```python
from build123d import *

# Parameters (mm, degrees)
SKETCH1_R           = 2.54
BOSS_EXTRUDE1_DEPTH = 3.175
FILLET1_R           = 6.35
CUT_EXTRUDE1_DEPTH  = 342.972704503
FILLET2_R           = 3.175
SKETCH3_R           = 2.54
CUT_EXTRUDE2_DEPTH  = 342.972704503
FILLET3_R           = 1.5875


with BuildPart() as part:
    # Sketch1 → Boss-Extrude1 (new body)
    with BuildSketch(Plane.XY):
        Polygon((0, 25.4), (0, 0), (127, 0), (127, 25.4), (152.4, 88.9), (317.5, 88.9), (317.5, 127), (279.4, 127), (152.4, 127), (40.64, 127), align=None)
        with Locations((12.7, 12.7)):
            Circle(SKETCH1_R, mode=Mode.SUBTRACT)
        with Locations((63.5, 12.7)):
            Circle(SKETCH1_R, mode=Mode.SUBTRACT)
        with Locations((114.3, 12.7)):
            Circle(SKETCH1_R, mode=Mode.SUBTRACT)
        Polygon((302.262821178, 101.346), (306.075642355, 107.95), (302.262821178, 114.554), (294.637178822, 114.554), (290.824357645, 107.95), (294.637178822, 101.346), align=None, mode=Mode.SUBTRACT)
    extrude(amount=BOSS_EXTRUDE1_DEPTH)

    # Fillet1
    fillet1_edges = [part.edges().sort_by_distance(p)[0] for p in [
        (40.64, 127, 1.5875),
        (317.5, 127, 1.5875),
        (317.5, 88.9, 1.5875),
        (152.4, 88.9, 1.5875),
        (127, 25.4, 1.5875),
        (127, 0, 1.5875),
        (0, 0, 1.5875),
        (0, 25.4, 1.5875),
    ]]
    fillet(fillet1_edges, radius=FILLET1_R)

    # Sketch2 → Cut-Extrude1 (cut, through all)
    with BuildSketch(Plane.XY.offset(3.175)):
        Polygon((49.23831861, 114.3), (13.67831861, 25.4), (39.597669611, 25.4), (75.157669611, 114.3), align=None)
        Polygon((86.100324499, 114.3), (50.540324499, 25.4), (76.459675501, 25.4), (112.019675501, 114.3), align=None)
        Polygon((122.962330389, 114.3), (87.402330389, 25.4), (113.32168139, 25.4), (148.88168139, 114.3), align=None)
    extrude(amount=-CUT_EXTRUDE1_DEPTH, mode=Mode.SUBTRACT)

    # Fillet2
    fillet2_edges = [part.edges().sort_by_distance(p)[0] for p in [
        (76.459675501, 25.4, 1.5875),
        (50.540324499, 25.4, 1.5875),
        (86.100324499, 114.3, 1.5875),
        (112.019675501, 114.3, 1.5875),
        (148.88168139, 114.3, 1.5875),
        (113.32168139, 25.4, 1.5875),
        (87.402330389, 25.4, 1.5875),
        (122.962330389, 114.3, 1.5875),
        (39.597669611, 25.4, 1.5875),
        (13.67831861, 25.4, 1.5875),
        (49.23831861, 114.3, 1.5875),
        (75.157669611, 114.3, 1.5875),
    ]]
    fillet(fillet2_edges, radius=FILLET2_R)

    # Sketch3 → Cut-Extrude2 (cut, through all)
    with BuildSketch(Plane.XY.offset(3.175)):
        with Locations((45.72, 120.65)):
            Circle(SKETCH3_R)
        with Locations((119.38, 120.65)):
            Circle(SKETCH3_R)
        with Locations((193.04, 120.65)):
            Circle(SKETCH3_R)
        with Locations((266.7, 120.65)):
            Circle(SKETCH3_R)
    extrude(amount=-CUT_EXTRUDE2_DEPTH, mode=Mode.SUBTRACT)

    # Fillet3
    fillet3_edges = [part.edges().sort_by_distance(p)[0] for p in [
        (294.637178822, 101.346, 1.5875),
        (302.262821178, 101.346, 1.5875),
        (306.075642355, 107.95, 1.5875),
        (302.262821178, 114.554, 1.5875),
        (294.637178822, 114.554, 1.5875),
        (290.824357645, 107.95, 1.5875),
    ]]
    fillet(fillet3_edges, radius=FILLET3_R)


solid = part.part
```
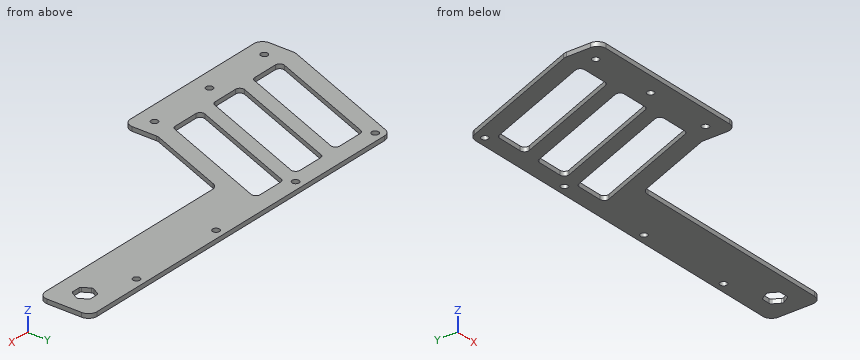
Verification items for the finished model (mm, model axes). Round coordinates to 2 decimals unless told otherwise and drop trailing zeros. Order: outer loops, then holes, each group sorted by start corner. A loop starts at its lowest first (then second) coordinate and runs counter-clockwise, first axis right, second up. Notation, with made-up numbers: (0, -35) - (18, -35) arc R23 ccw to (18, -20) - close; hole circle Ø9 at (37.25, 9). An arc over 180 degrees is marked (long way). Use CSV: the item, a comma, the result in double quotes.
(1) Gauge pin test, flat ends, axial feed: pin 1 Ø1.6 at (y, z) = (14.5, 2) entering from +X; pin 2 Ø3 at (x, y) = (266.7, 120.65) entering from -Z. Record the tip position at first contact, or that the pin passes through.
Entries:
pin 1,"x = 127"
pin 2,"through"
(2) Section check C-C on x = 283. Record the boundary of the cut face in (y, z) (3 decimals).
Entries:
outline,"(88.9, 0) - (127, 0) - (127, 3.175) - (88.9, 3.175) - close"
(3) Thickness scan on probe 1 along X at (y, z) = (60, 1.45); probe 2 along X at (y, z) = (98.5, 2.25); probe 3 along Y at (x, z) = (177, 2.4). Record the ranges inside material, lowest first. Write a range as from..to.
Entries:
probe 1,"13.84..27.52, 53.44..64.38, 90.3..101.24, 127.16..140.84"
probe 2,"29.24..42.92, 68.84..79.78, 105.7..116.64, 142.56..317.5"
probe 3,"88.9..127"
(4) Section check A-A on y = 66.5. Record the boundary of the cut face in (x, z) (3 decimals).
Entries:
outline,"(16.44, 0) - (30.118, 0) - (30.118, 3.175) - (16.44, 3.175) - close; (56.038, 0) - (66.98, 0) - (66.98, 3.175) - (56.038, 3.175) - close; (92.9, 0) - (103.842, 0) - (103.842, 3.175) - (92.9, 3.175) - close; (129.762, 0) - (143.44, 0) - (143.44, 3.175) - (129.762, 3.175) - close"
(5) Section check B-B on z = 1.85. State how many separate pieces and enclosed holes the cut face has, and give its area (3 significant figures).
Entries:
separate pieces,"1"
enclosed holes,"11"
area,"14,900 mm^2"
